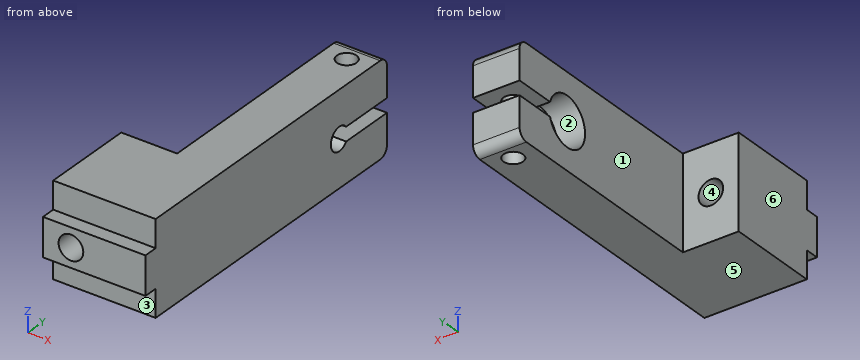
Autodesk Inventor part; units mm, degrees
ref_plane "YZ Plane" through (0, 0, 0) normal (1, 0, 0) x (0, 1, 0)
ref_plane "XZ Plane" through (0, 0, 0) normal (0, 1, 0) x (-1, 0, 0)
ref_plane "XY Plane" through (0, 0, 0) normal (0, 0, 1) x (1, 0, 0)
sketch "Sketch1" plane through (0, 0, 0) normal (0, 0, 1) x (1, 0, 0)
  line L0 (-26.4, 0) -> (4.4, 0) construction
  line L1 (0, -28.2297) -> (0, 100.056) construction
  line L2 (0, 0) -> (-22, 0)
  line L3 (-22, 0) -> (-22, 20)
  line L4 (-22, 20) -> (-10, 20)
  line L5 (-10, 20) -> (-10, 68)
  line L6 (-10, 68) -> (0, 68)
  line L7 (0, 68) -> (0, 0)
  dimension "d0" = 68
  dimension "d1" = 10
  dimension "d2" = 22
  dimension "d3" = 20
extrude "Extrusion1" add sketch "Sketch1" along normal mid plane 20
sketch "Sketch2" plane through (-22, 0, 10) normal (0, -1, 0) x (1, 0, 0)
  line L0 (-4.4, -10) -> (26.4, -10) construction
  line L1 (22, -24) -> (22, 4) construction
  line L2 (0, 0) -> (0, -20) construction
  line L3 (0, -5.9) -> (22, -5.9)
  line L4 (22, -5.9) -> (22, -14.1)
  line L5 (22, -14.1) -> (0, -14.1)
  line L6 (0, -14.1) -> (0, -5.9)
  point P0 (22, -10)
  point P1 (22, -10)
  dimension "d6" = 8.2
extrude "Extrusion2" add sketch "Sketch2" along normal blind 3
sketch "Sketch4" plane through (-22, 20, 10) normal (0, 1, 0) x (1, 0, 0)
  line L0 (-4.4, 10) -> (26.4, 10)
  line L1 (22, 24) -> (22, -4)
  point P0 (22, 10)
  point P1 (6, 10)
  dimension "d18" = 16
hole "Hole2" at (-16, 20, 0) direction (0, -1, 0) diameter 5.3 end through all
sketch "Esquisse5" plane through (-10, 20, -10) normal (-1, 0, 0) x (0, 0, 1)
  line L0 (10, -33.1749) -> (10, 52.2673)
  line L1 (5.9, -20) -> (0, -20)
  point P0 (10, -20)
  point P1 (10, 34)
  dimension "d28" = 54
hole "Perçage3" at (-10, 54, 0) direction (1, 0, 0) diameter 5 end through all
fillet "Congé2" radius 2 1 edges at (-5, 68, -10)
fillet "Congé3" radius 2 1 edges at (-5, 68, 10)
sketch "Esquisse6" plane through (-10, 20, -10) normal (-1, 0, 0) x (0, 0, 1)
  line L0 (10, -28.7649) -> (10, 59.9082)
  line L1 (5.9, -20) -> (0, -20)
  point P0 (10, -20)
  point P1 (10, 34)
  dimension "d38" = 54
hole "Perçage4" at (-10, 54, 0) direction (1, 0, 0) diameter 10.5 depth 6
sketch "Esquisse8" plane through (-10, 20, -10) normal (-1, 0, 0) x (0, 0, 1)
  line L0 (10, -28.9396) -> (10, 64.2926)
  line L1 (10, 34) -> (8.5, 34)
  line L2 (8.5, 34) -> (8.5, 50.8033)
  line L3 (8.5, 50.8033) -> (10, 50.8033)
  line L4 (5.9, -20) -> (0, -20)
  line L5 (20, 46) -> (20, 0)
  line L6 (10, 34) -> (10, 50.8033)
  point P0 (10, -20)
  dimension "d50" = 54
  dimension "d51" = 3
  dimension "d52" = 10
  dimension "d53" = 16.8033
  dimension "d54" = 8.9396
  dimension "d55" = 93.2322
extrude "Extrusion3" cut sketch "Esquisse8" against normal through all
mirror "Symétrie1" about plane through (-10, 70.8033, 0) normal (0, 0, -1) of "Extrusion3"
sketch "Esquisse9" plane through (0, 0, 10) normal (0, 0, 1) x (1, 0, 0)
  line L0 (-10, 66) -> (-10, 20)
  line L1 (-22, 0) -> (0, 0)
  point P0 (-5, 63)
  dimension "d58" = 5
  dimension "d59" = 63
hole "Perçage5" at (-5, 63, 10) direction (0, 0, -1) diameter 4.2 end through all
properties part number "P116SupportFibre" material "ABS"
Design review of the part built by this model. Coordinates are the model's own, in mm. Face numbers are marked on the shaded views. A direction names the side the tool comes from. Give positions to 0.01 mm unless a question says otherwise; leave off trailing zeros. Write each loop counter-clockwise with the first axis right and the second up, starting at its lowest first coordinate (ties: lowest second). Pieces come first, ordered by that corner, then holes.
(1) Clearance check with flat-ended pins moving along their axes: pin 1 Ø4 at (x, z) = (-16, 0) entering from +Y; pin 2 Ø3 at (x, z) = (-13, 8) entering from -Y; pin 3 Ø10 at (y, z) = (52, -2.5) entering from -X; pin 4 Ø3.5 at (x, z) = (-17.5, -4.5) entering from +Y. State where each tip first meets the part, or that it passes through.
Checked values:
pin 1: passes through
pin 2: stops at y = 0
pin 3: stops at x = -10
pin 4: stops at y = 20
(2) Add section D-D (z = 0.75). Give the boundary of the cut face in (x, y), and give its area (3 significant figures).
Checked values:
outline: (-22, -3) - (-18.54, -3) - (-18.54, 20) - (-22, 20) - close; (-13.46, -3) - (0, -3) - (0, 51.62) - (-4, 51.62) - (-4, 48.8) - (-10, 48.8) - (-10, 20) - (-13.46, 20) - close
area: 688 mm2
(3) Tool access review of the marked faces 1, 2 and 3: name each direction out of +Z, -Z, +X, -X, +Y, -Y from which nothing blocks a thin tool from reaching the whole face with its end or side.
Checked values:
face 1: +Z, -Z, -X, +Y
face 2: -X
face 3: -Z, +X, -X, -Y
(4) Add section B-B (x = -5). Give the boundary of the cut face in (y, z), and give its area (3 significant figures).
Checked values:
outline: (-3, -4.1) - (0, -4.1) - (0, -10) - (60.9, -10) - (60.9, -1.5) - (59.03, -1.5) arc R5.25 cw (long way) to (59.03, 1.5) - (60.9, 1.5) - (60.9, 10) - (0, 10) - (0, 4.1) - (-3, 4.1) - close; (65.1, -10) - (66, -10) arc R2 ccw to (68, -8) - (68, -1.5) - (65.1, -1.5) - close; (65.1, 1.5) - (68, 1.5) - (68, 8) arc R2 ccw to (66, 10) - (65.1, 10) - close
area: 1,200 mm2
(5) Mouldability with a two-part tool opening along X and no side actions: class the marked faces 4, 5 and 6 as +X half, -X half, draft (parallel to the pull), parting line (faces both ways), or undercut.
Checked values:
face 4: undercut
face 5: draft
face 6: -X half
(6) Wall thickness on line 1 along X through (y, z) = (63, -3.5); line 2 along Z through (x, y) = (-3, 64.5); line 3 along Y through (x, z) = (-7.25, -7.75): over which ranges is each line inside the solid? List them lowest first.
Checked values:
line 1: x = -10 to -7.1, -2.9 to 0
line 2: z = -10 to -1.5, 1.5 to 10
line 3: y = 0 to 68
(7) Add section C-C (y = 63). Give the boundary of the cut face in (x, z).
Checked values:
outline: (-10, -10) - (-7.1, -10) - (-7.1, -1.5) - (-10, -1.5) - close; (-10, 1.5) - (-7.1, 1.5) - (-7.1, 10) - (-10, 10) - close; (-2.9, -10) - (0, -10) - (0, -1.5) - (-2.9, -1.5) - close; (-2.9, 1.5) - (0, 1.5) - (0, 10) - (-2.9, 10) - close
(8) Add section A-A (y = 54). Give the boundary of the cut face in (x, z).
Checked values:
outline: (-10, -10) - (0, -10) - (0, -2.5) - (-4, -2.5) - (-4, -5.25) - (-10, -5.25) - close; (-10, 5.25) - (-4, 5.25) - (-4, 2.5) - (0, 2.5) - (0, 10) - (-10, 10) - close
